For this review, take the finished solid that the model builds, in its own axes (mm). A direction names the side the tool comes from. Give positions to 0.01 mm unless a question says otherwise; leave off trailing zeros. Write each loop counter-clockwise with the first axis right and the second up, starting at its lowest first coordinate (ties: lowest second). Pieces come first, ordered by that corner, then holes. Notation, with made-up numbers: (-37.5, -24.75) -> (-33.5, -24.75) arc R15 ccw to (-33.5, -20.75) -> close; hole circle Ø10 at (35, 56.5). An arc over 180 degrees is marked (long way). Answer as CSV lines item,"result".
```python
from build123d import *

# Parameters (mm, degrees)
BOSS_EXTRU_1_DEPTH      = 10
ESQUISSE2_R             = 2
ENL_V_MAT_EXTRU_1_DEPTH = 22.552262062
CONG_1_R                = 5
ESQUISSE3_R             = 2
ENL_V_MAT_EXTRU_2_DEPTH = 19.716636984
CONG_2_R                = 5


with BuildPart() as part:
    # Esquisse1 → Boss.-Extru.1 (new body)
    with BuildSketch(Plane(origin=(0, 0, 0), x_dir=(0, 0, -1), z_dir=(1, 0, 0))):
        Polygon((6.75, 0), (-6.75, 0), (-6.75, 13.5), (-8.25, 13.5), (-8.25, -1.5), (6.75, -1.5), align=None)
    extrude(amount=BOSS_EXTRU_1_DEPTH)

    # Esquisse2 → Enlèv. mat.-Extru.1 (cut, through all)
    with BuildSketch(Plane(origin=(0, 0, 6.75), x_dir=(-1, 0, 0), z_dir=(0, 0, -1))):
        with Locations(Location((-5, 6.5, 0), (0, 0, 90))):
            Circle(ESQUISSE2_R)
    extrude(amount=-ENL_V_MAT_EXTRU_1_DEPTH, mode=Mode.SUBTRACT)

    # Congé1
    cong_1_edges = [part.edges().sort_by_distance(p)[0] for p in [
        (0, 13.5, 7.5),
        (10, 13.5, 7.5),
    ]]
    fillet(cong_1_edges, radius=CONG_1_R - 0.0001)  # a hair under: the kernel refuses the full size

    # Esquisse3 → Enlèv. mat.-Extru.2 (cut, through all)
    with BuildSketch(Plane(origin=(0, 0, 0), x_dir=(1, 0, 0), z_dir=(0, 1, 0))):
        with Locations(Location((5, 0, 0), (0, 0, 270))):
            Circle(ESQUISSE3_R)
    extrude(amount=-ENL_V_MAT_EXTRU_2_DEPTH, mode=Mode.SUBTRACT)

    # Congé2
    cong_2_edges = [part.edges().sort_by_distance(p)[0] for p in [
        (10, -0.75, -6.75),
        (0, -0.75, -6.75),
    ]]
    fillet(cong_2_edges, radius=CONG_2_R - 0.0001)  # a hair under: the kernel refuses the full size


solid = part.part
```
Q1. Add section D-D (z = 3). Write out the cut boundary in (x, y).
Answer block:
outline,"(0, -1.5) -> (10, -1.5) -> (10, 0) -> (0, 0) -> close"
Q2. To check wall thickness, follow probe 1 along X at (y, z) = (6.5, 7.4); probe 2 along Z at (x, y) = (2.25, 12.5); probe 3 along Y at (x, z) = (4.5, 4). State the ranges of each line that lie inside material, in increasing order. Write a range as [from, to].
Answer block:
probe 1,"x = [0, 3], [7, 10]"
probe 2,"z = [6.75, 8.25]"
probe 3,"y = [-1.5, 0]"
Q3. Clearance check with flat-ended pins moving along their axes: pin 1 (2.5 mm diameter, centred on x = 5, z = 0, fed in from +Y); pin 2 (3 mm diameter, centred on x = 5.5, z = -0.5, fed in from +Y); pin 3 (4 mm diameter, centred on y = 4, z = 5.5, fed in from -X); pin 4 (2 mm diameter, centred on x = 1.5, y = 4, fed in from -Z). State where each tip first meets the part, or that it passes through.
Answer block:
pin 1,"passes through"
pin 2,"stops at y = 0"
pin 3,"stops at x = 0"
pin 4,"stops at z = 6.75"
Q4. For faces 1 (the flat face through (2.7, 6.7, 6.75)), 2 (the cylindrical face through (1.43, 12, 7.51)), list the 3-axis set-ups (+Z, -Z, +X, -X, +Y, -Y) from which the entire face can be reached by the end or side of a thin tool; tool diameter is ignored.
Answer block:
face 1,"-Z, +X, -X, +Y"
face 2,"+Z, -Z, -X, +Y"
Q5. Add section C-C (x = 6.75). Write out the cut boundary in (y, z).
Answer block:
outline,"(-1.5, -6.43) -> (0, -6.43) -> (0, -0.97) -> (-1.5, -0.97) -> close; (-1.5, 0.97) -> (0, 0.97) -> (0, 6.75) -> (5.53, 6.75) -> (5.53, 8.25) -> (-1.5, 8.25) -> close; (7.47, 6.75) -> (13.18, 6.75) -> (13.18, 8.25) -> (7.47, 8.25) -> close"
Q6. Draft analysis for pull direction Y (two halves, no side actions). For faces 3 (the flat face through (2.7, 0, -0.1)), 4 (the cylindrical face through (6.352, 5.026, 7.49)), 5 (the cylindrical face through (7, -1, 0)), state which applies: released by +Y, released by -Y, zero draft, split by the parting line, or undercut.
Answer block:
face 3,"released by +Y"
face 4,"undercut"
face 5,"zero draft"
Q7. Add section B-B (y = 6.5). Write out the cut boundary in (x, z).
Answer block:
outline,"(0, 6.75) -> (3, 6.75) -> (3, 8.25) -> (0, 8.25) -> close; (7, 6.75) -> (10, 6.75) -> (10, 8.25) -> (7, 8.25) -> close"
Q8. Add section A-A (z = -0.25). Write out the cut boundary in (x, y).
Answer block:
outline,"(0, -1.5) -> (3.02, -1.5) -> (3.02, 0) -> (0, 0) -> close; (6.98, -1.5) -> (10, -1.5) -> (10, 0) -> (6.98, 0) -> close"
